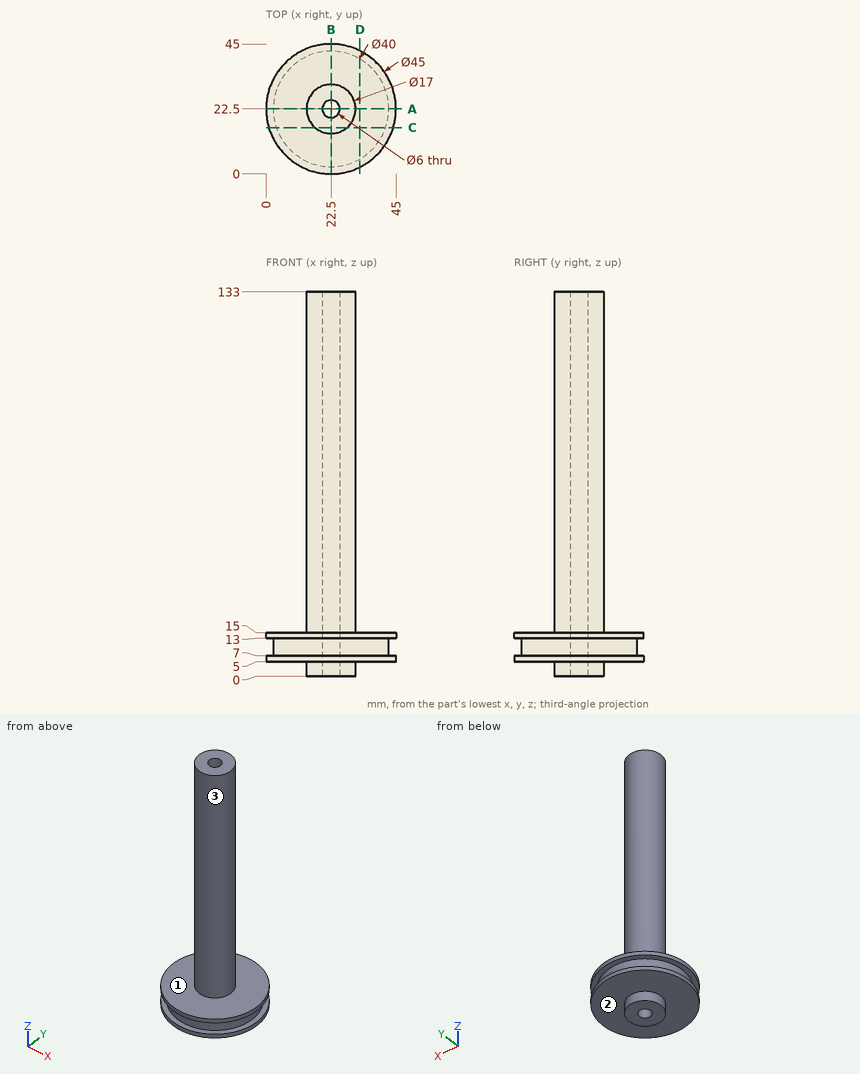
Print and shaded views of the part. All mm, measured from the part's lowest x, y and z. Give positions to 0.01 mm unless a question says otherwise; leave off trailing zeros. Loops run counter-clockwise (first coordinate to the right, second up) from the corner with the lowest first, then second, coordinate; pieces in that order, holes last. Notation, with made-up numbers: (85.25, -33) - (108.25, -33) arc R25 cw to (108.25, -12) - close; hole circle Ø1 at (83.5, 68.5). An arc over 180 degrees is marked (long way). Use a Markdown table: item, result.
(1) Wall check: line 1 along Z through (x, y) = (41.5, 13); line 2 along Z through (x, y) = (35, 15); line 3 along Y through (x, z) = (21.5, 62). Give the ranges that are in metal, low to high.
Taken from the geometry:
| item | result |
|---|---|
| line 1 | 5 to 7, 13 to 15 |
| line 2 | 5 to 15 |
| line 3 | 14.06 to 19.67, 25.33 to 30.94 |
(2) Band-saw the part on A-A (y = 22.5). Give the cut face in (x, z), and give its area (3 significant figures).
Taken from the geometry:
| item | result |
|---|---|
| outline | (0, 5) - (14, 5) - (14, 0) - (19.5, 0) - (19.5, 133) - (14, 133) - (14, 15) - (0, 15) - (0, 13) - (2.5, 13) - (2.5, 7) - (0, 7) - close; (25.5, 0) - (31, 0) - (31, 5) - (45, 5) - (45, 7) - (42.5, 7) - (42.5, 13) - (45, 13) - (45, 15) - (31, 15) - (31, 133) - (25.5, 133) - close |
| area | 1,710 mm2 |
(3) Drop flat-ended pins along their axis: pin 1 Ø8 at (x, z) = (21.5, 108.5) entering from -Y; pin 2 Ø5 at (x, y) = (9.5, 24.5) entering from -Z; pin 3 Ø6 at (x, z) = (28.5, 71.5) entering from -Y. Give the stop position or say it passes through.
Taken from the geometry:
| item | result |
|---|---|
| pin 1 | y = 14 |
| pin 2 | z = 5 |
| pin 3 | y = 14.55 |
(4) Pull direction Z, two halves, no side cores. Call the marked faces 1, 2 and 3: +Z half, -Z half, draft (parallel to the pull), parting line (faces both ways), or undercut.
Taken from the geometry:
| item | result |
|---|---|
| face 1 | +Z half |
| face 2 | -Z half |
| face 3 | draft |
(5) Band-saw the part on D-D (x = 32.5). Give the cut face in (y, z), and give its area (3 significant figures).
Taken from the geometry:
| item | result |
|---|---|
| outline | (2.34, 5) - (42.66, 5) - (42.66, 7) - (39.82, 7) - (39.82, 13) - (42.66, 13) - (42.66, 15) - (2.34, 15) - (2.34, 13) - (5.18, 13) - (5.18, 7) - (2.34, 7) - close |
| area | 369 mm2 |
(6) Band-saw the part on C-C (y = 16). Give the cut face in (x, z), and give its area (3 significant figures).
Taken from the geometry:
| item | result |
|---|---|
| outline | (0.96, 5) - (17.02, 5) - (17.02, 0) - (27.98, 0) - (27.98, 5) - (44.04, 5) - (44.04, 7) - (41.41, 7) - (41.41, 13) - (44.04, 13) - (44.04, 15) - (27.98, 15) - (27.98, 133) - (17.02, 133) - (17.02, 15) - (0.96, 15) - (0.96, 13) - (3.59, 13) - (3.59, 7) - (0.96, 7) - close |
| area | 1,750 mm2 |
